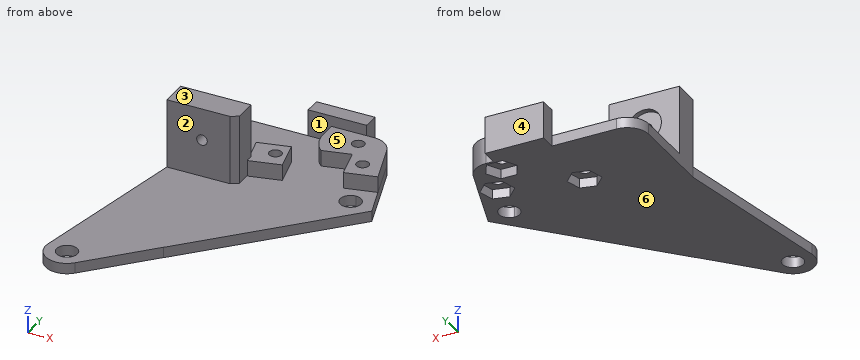
from build123d import *

# Parameters (mm, degrees)
SKETCH2_R                = 3.81
BOSS_EXTRUDE1_DEPTH      = 2.54
SKETCH5_W                = 16.764
SKETCH5_H                = 6.35
BOSS_EXTRUDE2_DEPTH      = 16.51
SKETCH6_R                = 4.1275
CUT_EXTRUDE2_DEPTH       = 1.27
SKETCH7_R                = 1.27
CUT_EXTRUDE3_DEPTH       = 65.77
CUT_EXTRUDE4_DEPTH       = 2.286
BOSS_EXTRUDE3_DEPTH      = 3.81
F_4_CLEARANCE_HOLE1_D    = 2.9464
SKETCH14_W               = 13.97
SKETCH14_H               = 3.81
BOSS_EXTRUDE6_DEPTH      = 6.35
BOSS_EXTRUDE6_DEPTH_BACK = 2.54
FILLET1_R                = 5.08
CUT_EXTRUDE5_DEPTH       = 17.51
CUT_EXTRUDE5_DEPTH_BACK  = 3.54
SKETCH19_R               = 2.4892
BOSS_EXTRUDE8_DEPTH      = 2.54
CUT_EXTRUDE8_DEPTH       = 2.54


with BuildPart() as part:
    # Sketch2 → Boss-Extrude1 (new body)
    with BuildSketch(Plane.XY):
        with BuildLine():
            Line((-17.068825413, -8.459178389), (-41.402, 40.64))
            Line((-41.402, 40.64), (-41.402, 66.04))
            Line((-41.402, 66.04), (-1.524, 66.04))
            Line((-1.524, 66.04), (18.109053667, 5.913093546))
            ThreePointArc((18.109053667, 5.913093546), (7.204933647, -17.634949139), (-17.068825413, -8.459178389))
        make_face()
        Circle(SKETCH2_R, mode=Mode.SUBTRACT)
    extrude(amount=BOSS_EXTRUDE1_DEPTH)

    # Sketch5 → Boss-Extrude2 (add)
    with BuildSketch(Plane.XY.offset(2.54)):
        with Locations((-33.02, 43.815)):
            Rectangle(SKETCH5_W, SKETCH5_H)
    extrude(amount=BOSS_EXTRUDE2_DEPTH)

    # Sketch6 → Cut-Extrude2 (cut)
    with BuildSketch(Plane(origin=(0, 46.99, 0), x_dir=(1, 0, 0), z_dir=(0, 1, 0))):
        with Locations((-33.02, -11.43)):
            Circle(SKETCH6_R)
    extrude(amount=-CUT_EXTRUDE2_DEPTH, mode=Mode.SUBTRACT)

    # Sketch7 → Cut-Extrude3 (cut, through all)
    with BuildSketch(Plane(origin=(0, 45.72, 0), x_dir=(1, 0, 0), z_dir=(0, 1, 0))):
        with Locations((-33.02, -11.43)):
            Circle(SKETCH7_R)
    extrude(amount=-CUT_EXTRUDE3_DEPTH, mode=Mode.SUBTRACT)

    # Sketch9 → Cut-Extrude4 (cut)
    with BuildSketch(Plane(origin=(0, 0, 0), x_dir=(-1, 0, 0), z_dir=(0, 0, -1))):
        Polygon((3.171122265, 62.23), (5.077532854, 58.928), (8.890354032, 58.928), (10.796764621, 62.23), (8.890354032, 65.532), (5.077532854, 65.532), align=None)
        Polygon((24.379877895, 49.663956202), (23.308143816, 53.323053276), (19.603405755, 54.224452874), (16.970401774, 51.466755398), (18.042135853, 47.807658324), (21.746873914, 46.906258726), align=None)
        Polygon((5.918476139, 54.15579827), (4.846742059, 57.814895344), (1.142003999, 58.716294942), (-1.490999983, 55.958597466), (-0.419265903, 52.299500392), (3.285472157, 51.398100794), align=None)
    extrude(amount=-CUT_EXTRUDE4_DEPTH, mode=Mode.SUBTRACT)

    # Sketch8 → Boss-Extrude3 (add)
    with BuildSketch(Plane.XY.offset(2.54)):
        with BuildLine():
            Line((-15.367, 66.04), (-6.983943443, 66.04))
            Line((-6.983943443, 66.04), (-1.524, 66.04))
            Line((-1.524, 66.04), (3.09175139, 51.904101595))
            Line((3.09175139, 51.904101595), (-4.240438106, 50.120107003))
            Line((-4.240438106, 50.120107003), (-6.088713216, 57.716488409))
            Line((-6.088713216, 57.716488409), (-12.708473154, 56.10583501))
            ThreePointArc((-12.708473154, 56.10583501), (-14.673699407, 58.891843255), (-15.367, 62.23))
            Line((-15.367, 62.23), (-15.367, 66.04))
        make_face()
        Polygon((-17.142042414, 46.981018422), (-18.990317524, 54.577399829), (-26.415687706, 52.770733449), (-24.567412596, 45.174352043), align=None)
    extrude(amount=BOSS_EXTRUDE3_DEPTH)

    # #4 Clearance Hole1 (through all)
    with Locations(Plane.XY.offset(6.35)):
        with Locations((-6.983943443, 62.23), (-20.675139834, 50.5653558), (-2.213738078, 55.057197868)):
            Hole(F_4_CLEARANCE_HOLE1_D / 2)

    # Sketch14 → Boss-Extrude6 (add, two sides)
    with BuildSketch(Plane.XY.offset(2.54)) as boss_extrude6_sk:
        with Locations((-13.968943443, 67.945)):
            Rectangle(SKETCH14_W, SKETCH14_H)
    extrude(amount=BOSS_EXTRUDE6_DEPTH)
    extrude(boss_extrude6_sk.sketch, amount=-BOSS_EXTRUDE6_DEPTH_BACK)

    # Fillet1
    fillet1_edges = [part.edges().sort_by_distance(p)[0] for p in [
        (-41.402, 66.04, 1.27),
        (-1.524, 66.04, 3.175),
    ]]
    fillet(fillet1_edges, radius=FILLET1_R)

    # Sketch15 → Cut-Extrude5 (cut, two sides)
    with BuildSketch(Plane.XY.offset(2.54)) as cut_extrude5_sk:
        with BuildLine():
            ThreePointArc((-0.315167053, 48.411374113), (-18.310138041, 44.816284079), (-33.674369734, 34.782140486))
            ThreePointArc((-33.674369734, 34.782140486), (-33.731327517, 31.262340905), (-30.211527936, 31.205383122))
            ThreePointArc((-30.211527936, 31.205383122), (-16.427248714, 40.207684038), (-0.28275743, 43.433079608))
            ThreePointArc((-0.28275743, 43.433079608), (2.190185011, 45.938431672), (-0.315167053, 48.411374113))
        make_face()
    extrude(amount=CUT_EXTRUDE5_DEPTH, mode=Mode.SUBTRACT)
    extrude(cut_extrude5_sk.sketch, amount=-CUT_EXTRUDE5_DEPTH_BACK, mode=Mode.SUBTRACT)

    # Sketch19 → Boss-Extrude8 (add, through all)
    with BuildSketch(Plane.XY.offset(2.54)):
        with BuildLine():
            Line((5.466200245, 44.632269783), (-40.158007355, -3.769954845))
            ThreePointArc((-40.158007355, -3.769954845), (-46.15516131, -4.814733016), (-48.848797168, 0.64436424))
            Line((-48.848797168, 0.64436424), (-41.402, 40.64))
            Line((-41.402, 40.64), (3.09175139, 51.904101595))
            Line((3.09175139, 51.904101595), (5.466200245, 44.632269783))
        make_face()
        with Locations((-0.298962241, 45.92222686)):
            Circle(SKETCH19_R, mode=Mode.SUBTRACT)
        with Locations((-43.854625645, -0.285501773)):
            Circle(SKETCH19_R, mode=Mode.SUBTRACT)
    extrude(amount=-BOSS_EXTRUDE8_DEPTH)

    # Sketch20 → Cut-Extrude8 (cut)
    with BuildSketch(Plane.XY.offset(2.54)):
        Polygon((-40.158007355, -3.769954845), (10.729493517, 49.863783044), (48.07174347, 14.433588323), (-7.673080914, -44.319607422), align=None)
    extrude(amount=-CUT_EXTRUDE8_DEPTH, mode=Mode.SUBTRACT)


solid = part.part
Design review of the part built by this model. Coordinates are the model's own, in mm. Face numbers are marked on the shaded views. A direction names the side the tool comes from. Coordinates: 2 decimals unless noted, no trailing zeros. Loops run counter-clockwise (first coordinate to the right, second up) from the corner with the lowest first, then second, coordinate; pieces in that order, holes last.
Item 1: For the marked faces 5 and 6, list the 3-axis set-ups (+Z, -Z, +X, -X, +Y, -Y) from which the entire face can be reached by the end or side of a thin tool; tool diameter is ignored.
Completed:
face 5: +Z, +X, -X, -Y
face 6: -Z, +X, -X, +Y, -Y
Item 2: Add section D-D (y = 16.5). Write out the cut boundary in (x, z).
Completed:
outline: (-45.9, 0) - (-20.93, 0) - (-20.93, 2.54) - (-45.9, 2.54) - close
Item 3: Wall thickness on L1, parallel to Z at x = -33.02, y = 46.35; L2, parallel to X at y = 46.6, z = 11.43; L3, parallel to Z at x = -33.02, y = 43.8: over which ranges is each line inside the solid? List them lowest first.
Completed:
L1: z = 0 to 7.3, 15.56 to 19.05
L2: x = -41.4 to -37.15, -28.89 to -24.64
L3: z = 0 to 10.16, 12.7 to 19.05
Item 4: Add section A-A (z = 11.43). Write out the cut boundary in (x, y), and give its area (3 significant figures).
Completed:
outline: (-41.4, 40.64) - (-34.29, 40.64) - (-34.29, 45.72) - (-37.15, 45.72) - (-37.15, 46.99) - (-41.4, 46.99) - close; (-31.75, 40.64) - (-26.31, 40.64) arc R48.41 cw to (-24.64, 41.67) - (-24.64, 46.99) - (-28.89, 46.99) - (-28.89, 45.72) - (-31.75, 45.72) - close
area: 82.2 mm2
Item 5: Draft analysis for pull direction Y (two halves, no side actions). For the marked faces 1, 2, 3 and 4, state which applies: pulls with the +Y half, pulls with the -Y half, needs draft (parallel to the pull), parting line crosses it, or undercut.
Completed:
face 1: undercut
face 2: pulls with the -Y half
face 3: needs draft
face 4: pulls with the +Y half
Item 6: Clearance check with flat-ended pins moving along their axes: pin 1 (5 mm diameter, centred on x = -33.02, z = 11.43, fed in from -Y); pin 2 (9 mm diameter, centred on x = -31, z = 12.5, fed in from +Y); pin 3 (4.5 mm diameter, centred on x = -6.98, y = 62.23, fed in from +Z); pin 4 (8 mm diameter, centred on x = -20, y = 49, fed in from -Z). State where each tip first meets the part, or that it passes through.
Completed:
pin 1: stops at y = 40.64
pin 2: stops at y = 46.99
pin 3: stops at z = 6.35
pin 4: stops at z = 0
Item 7: Add section B-B (x = -33.02). Write out the cut boundary in (y, z), and give its area (3 significant figures).
Completed:
outline: (3.8, 0) - (66.04, 0) - (66.04, 2.54) - (46.99, 2.54) - (46.99, 7.3) - (45.72, 7.3) - (45.72, 10.16) - (40.64, 10.16) - (40.64, 2.54) - (3.8, 2.54) - close; (40.64, 12.7) - (45.72, 12.7) - (45.72, 15.56) - (46.99, 15.56) - (46.99, 19.05) - (40.64, 19.05) - close
area: 240 mm2
Item 8: Add section C-C (x = -43). Write out the cut boundary in (y, z).
Completed:
outline: (-5.29, 0) - (-2.62, 0) - (-2.62, 2.54) - (-5.29, 2.54) - close; (2.05, 0) - (32.06, 0) - (32.06, 2.54) - (2.05, 2.54) - close
